Input: part model. Units: mm. Frame: model coordinates. Face numbers are marked on the shaded views. A direction names the side the tool comes from. Give positions to 0.01 mm unless a question says otherwise; leave off trailing zeros. Loops run counter-clockwise (first coordinate to the right, second up) from the corner with the lowest first, then second, coordinate; pieces in that order, holes last.
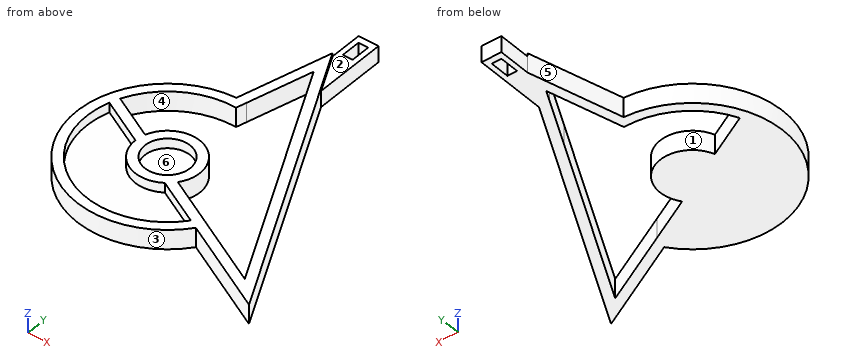
from build123d import *

# Parameters (mm, degrees)
F0_R     = 3.5
F1_DEPTH = 3
F2_DEPTH = 1.5
F3_DEPTH = 2.5
F4_W     = 1.5
F4_H     = 3
F5_DEPTH = 25
F6_ANGLE = 90


with BuildPart() as f1:
    # F0 (on Front) → F1 (new body)
    with BuildSketch(Plane.XZ):
        with BuildLine():
            ThreePointArc((5.0689673904, 14.5063923622), (-18.497586517, 12.604527099), (-6.7371360863, -7.9062349594))
            Line((-6.7371360863, -7.9062349594), (-3.0749836005, -21.8287352473))
            Line((-3.0749836005, -21.8287352473), (0, -15.8073518255))
            Line((0, -15.8073518255), (19.2700356521, 21.9269220071))
            Line((19.2700356521, 21.9269220071), (5.0689673904, 14.5063923622))
        make_face()
        with BuildLine():
            ThreePointArc((-5.5799534775, -6.4089575685), (-12.6983133538, -4.5436790019), (-17.5337629503, 1.0032786019))
            Line((-17.5337629503, 1.0032786019), (-10.852955333, 4.494222386))
            ThreePointArc((-10.852955333, 4.494222386), (-3.7954106953, 1.6482764037), (-2.1015582996, 9.067117884))
            Line((-2.1015582996, 9.067117884), (4.5792493177, 12.5580616681))
            Line((4.5792493177, 12.5580616681), (15.7938726924, 18.418074709))
            Line((15.7938726924, 18.418074709), (2.0825346023, -8.431246976))
            Line((2.0825346023, -8.431246976), (-1.7794150282, -15.9936546184))
            Line((-1.7794150282, -15.9936546184), (-2.6238568394, -17.6472269892))
            Line((-2.6238568394, -17.6472269892), (-5.1903976779, -7.8899419766))
            Line((-5.1903976779, -7.8899419766), (-5.5799534775, -6.4089575685))
        make_face(mode=Mode.SUBTRACT)
        with Locations((-6.1110062525, 6.0797566548)):
            Circle(F0_R, mode=Mode.SUBTRACT)
        with BuildLine():
            Line((-11.1109284274, 6.0518596218), (-18.0629985994, 2.4191721469))
            ThreePointArc((-18.0629985994, 2.4191721469), (-11.8999951454, 17.1584572825), (3.7191276324, 13.8010562737))
            Line((3.7191276324, 13.8010562737), (-3.2329425395, 10.1683687988))
            ThreePointArc((-3.2329425395, 10.1683687988), (-8.4266018096, 10.5112369059), (-11.1109284274, 6.0518596218))
        make_face(mode=Mode.SUBTRACT)
    extrude(amount=-F1_DEPTH)

    # F0 (on Front) → F2 (join)
    with BuildSketch(Plane.XZ):
        with BuildLine():
            ThreePointArc((3.7191276324, 13.8010562737), (-11.8999951454, 17.1584572825), (-18.0629985994, 2.4191721469))
            Line((-18.0629985994, 2.4191721469), (-11.1109284274, 6.0518596218))
            ThreePointArc((-11.1109284274, 6.0518596218), (-8.4266018096, 10.5112369059), (-3.2329425395, 10.1683687988))
            Line((-3.2329425395, 10.1683687988), (3.7191276324, 13.8010562737))
        make_face()
        with Locations((-6.1110062525, 6.0797566548)):
            Circle(F0_R)
    extrude(amount=-F2_DEPTH)

    # F0 (on Front) → F3 (join)
    with BuildSketch(Plane.XZ):
        Polygon((0, -15.8073518255), (-3.0749836005, -21.8287352473), (-3.0749836005, -26.8287352473), (0, -26.8287352473), align=None)
    extrude(amount=-F3_DEPTH)

    # F4 (on face) → F5 (cut)
    with BuildSketch(Plane(origin=(0, 2.5, 0), x_dir=(-1, 0, 0), z_dir=(0, 1, 0))):
        with Locations((1.5374918003, -24.3287352473)):
            Rectangle(F4_W, F4_H)
    extrude(amount=-F5_DEPTH, mode=Mode.SUBTRACT)


with BuildPart() as f1_1:
    # F6: moved
    add(f1.part.rotate(Axis((-1.5374918003, 0, -26.8287352473), (1, 0, 0)), F6_ANGLE))


solid = f1_1.part
(1) Pin query (flat end, axial travel): pin 1 Ø1 at (x, y) = (8, -22) entering from +Z; pin 2 Ø0.7 at (x, z) = (-1.5, -25.5) entering from -Y; pin 3 Ø0.8 at (y, z) = (-2.5, -26) entering from -X (3 decimals); pin 4 Ø0.8 at (y, z) = (-7, -25.5) entering from +X. Return the tip coordinate at first contact, or that it passes through.
Values follow:
pin 1: passes through
pin 2: stops at y = -46.24
pin 3: stops at x = -3.075
pin 4: stops at x = 0
(2) Ray query, probe 1 along X at (y, z) = (-3, -25.3); probe 2 along X at (y, z) = (-42, -25.9); probe 3 along Y at (x, z) = (-16.5, -25.2). Return the intervals inside material, ascending.
Values follow:
probe 1: x = -3.07 to -2.29, -0.79 to 0
probe 2: x = -16.76 to 4.54, 6.34 to 9.58, 14.14 to 15.82
probe 3: y = -42.29 to -39.86, -30.06 to -28.37, -25.96 to -23.52
(3) Reachability of the marked faces 4, 5 and 6 from +Z, -Z, +X, -X, +Y, -Y: full face, straight path, thin tool, end or side. Return the list, or none.
Values follow:
face 4: +Z, -Z
face 5: +Z, -Z, -X, +Y
face 6: +Z
(4) Cut plane D-D (y = -26). Return the cut outline in (x, z).
Values follow:
outline: (-18.29, -26.83) - (-16.53, -26.83) - (-16.53, -23.83) - (-18.29, -23.83) - close; (5.96, -26.83) - (7.65, -26.83) - (7.65, -23.83) - (5.96, -23.83) - close
(5) Cut plane B-B (z = -25.8). Return the cut outline in (x, y), and give its area (3 significant figures).
Values follow:
outline: (-6.74, -18.92) arc R14 ccw (long way) to (5.07, -41.34) - (19.27, -48.76) - (0, -11.02) - (0, 0) - (-3.07, 0) - (-3.07, -5) - close; hole (-17.53, -27.83) - (-10.85, -31.32) arc R5 cw (long way) to (-2.1, -35.9) - (15.79, -45.25) - (-2.62, -9.18) - (-5.58, -20.42) arc R12.5 ccw to start; hole (-2.29, -4) - (-0.79, -4) - (-0.79, -1) - (-2.29, -1) - close
area: 483 mm2
(6) Cut plane C-C (y = -43). Return the cut outline in (x, z), and give its area (3 significant figures).
Values follow:
outline: (-15.81, -26.83) - (3.59, -26.83) - (3.59, -23.83) - (1.27, -23.83) - (1.27, -25.33) - (-13.49, -25.33) - (-13.49, -23.83) - (-15.81, -23.83) - close; (8.26, -26.83) - (11.49, -26.83) - (11.49, -23.83) - (8.26, -23.83) - close; (14.65, -26.83) - (16.33, -26.83) - (16.33, -23.83) - (14.65, -23.83) - close
area: 50.9 mm2
(7) Cut plane A-A (y = -3). Return the cut outline in (x, z), and give its area (3 significant figures).
Values follow:
outline: (-3.07, -26.83) - (-2.29, -26.83) - (-2.29, -24.33) - (-3.07, -24.33) - close; (-0.79, -26.83) - (0, -26.83) - (0, -24.33) - (-0.79, -24.33) - close
area: 3.94 mm2
(8) Mould query, pull axis Y, two halves, no side actions, for the marked faces 1, 2 and 3. Classes: +Y half, -Y half, draft (parallel to the pull), parting line (faces both ways), or undercut.
Values follow:
face 1: undercut
face 2: draft
face 3: parting line
